```python
from build123d import *

# Parameters (mm, degrees)
F1_DEPTH      = 38.1
F1_DEPTH_BACK = 38.1
F2_R          = 5.08
F3_R          = 2.54
F4_R          = 11.1125
F5_DEPTH      = 25.4


with BuildPart() as f1:
    # F0 (on Front) → F1 (new body, two sides)
    with BuildSketch(Plane.XZ) as f1_sk:
        Polygon((-6.35, 0), (0, 0), (0, 69.85), (95.25, 69.85), (95.25, 76.2), (-6.35, 76.2), align=None)
    extrude(amount=F1_DEPTH)
    extrude(f1_sk.sketch, amount=-F1_DEPTH_BACK)

    # F2
    f2_edges = [f1.edges().sort_by_distance(p)[0] for p in [
        (-6.35, 0, 76.2),
    ]]
    fillet(f2_edges, radius=F2_R)

    # F3
    f3_edges = [f1.edges().sort_by_distance(p)[0] for p in [
        (0, 0, 69.85),
    ]]
    fillet(f3_edges, radius=F3_R)

    # F4 (on face) → F5 (cut)
    with BuildSketch(Plane.XY.offset(76.2)):
        with Locations((50.8, 0)):
            Circle(F4_R)
    extrude(amount=-F5_DEPTH, mode=Mode.SUBTRACT)


solid = f1.part
```
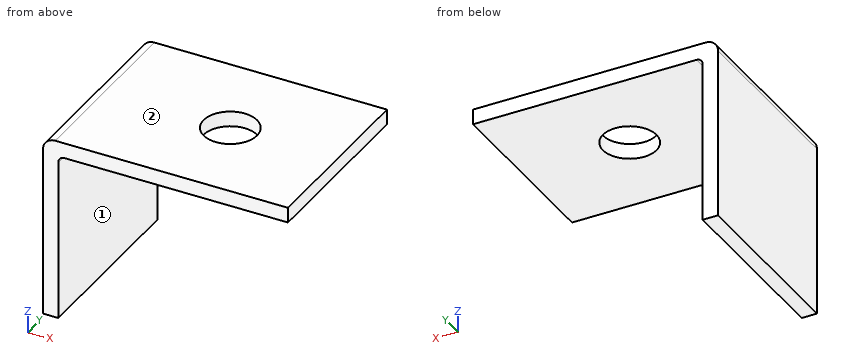
Could you check a few things on this model? Use its own coordinates, in mm. Face numbers are marked on the shaded views. A direction names the side the tool comes from. Round coordinates to 2 decimals unless told otherwise and drop trailing zeros. Loops run counter-clockwise (first coordinate to the right, second up) from the corner with the lowest first, then second, coordinate; pieces in that order, holes last. Notation, with made-up numbers: M 56.5,80.5 L 78.5,80.5 A16 cw 78.5,87.5 Z; hole C 88,48.5 d1. An arc over 180 degrees is marked long. Write item = value, one per line.
1. I want a section at D-D, the plane z = 51. Write out the boundary of the cut face in (x, y), and give its area (3 significant figures).
Results below:
outline = M -6.35,-38.1 L 0,-38.1 L 0,38.1 L -6.35,38.1 Z
area = 484 mm²
2. I want a section at B-B, the plane x = 50.8. Write out the boundary of the cut face in (y, z), and give its area (3 significant figures).
Results below:
outline = M -38.1,69.85 L -11.11,69.85 L -11.11,76.2 L -38.1,76.2 Z; M 11.11,69.85 L 38.1,69.85 L 38.1,76.2 L 11.11,76.2 Z
area = 343 mm²
3. I want a section at A-A, the plane y = 0. Write out the boundary of the cut face in (x, z).
Results below:
outline = M -6.35,0 L 0,0 L 0,67.31 A2.54 cw 2.54,69.85 L 39.69,69.85 L 39.69,76.2 L -1.27,76.2 A5.08 ccw -6.35,71.12 Z; M 61.91,69.85 L 95.25,69.85 L 95.25,76.2 L 61.91,76.2 Z
4. I want a section at C-C, the plane y = 15. Write out the boundary of the cut face in (x, z).
Results below:
outline = M -6.35,0 L 0,0 L 0,67.31 A2.54 cw 2.54,69.85 L 95.25,69.85 L 95.25,76.2 L -1.27,76.2 A5.08 ccw -6.35,71.12 Z
5. I need wall thicknesses on probe 1 along Y at (x, z) = (50.8, 72.25); probe 2 along Y at (x, z) = (42.5, 72); probe 3 along Z at (x, y) = (49.5, -28.5). Which ranges of each line are inside material? Lowest first, please.
Results below:
probe_1 = -38.1 to -11.11, 11.11 to 38.1
probe_2 = -38.1 to -7.39, 7.39 to 38.1
probe_3 = 69.85 to 76.2
6. Will this pin go through, and if not, where does the flat tip stop? P1, Ø6, axis at x = 71.5, y = -24, coming from the -Z side.
Results below:
P1 = 69.85
7. Which directions (+Z, -Z, +X, -X, +Y, -Y) give clear straight access to the entire face, cutting with the end or side of a thin tool? Please do the marked faces 1 and 2.
Results below:
face_1 = -Z, +X, +Y, -Y
face_2 = +Z, +X, -X, +Y, -Y
